Source: CAD feature listing. Evaluate the final solid. Frame: model axes, mm. A direction names the side the tool comes from. Coordinates: 2 decimals unless noted, no trailing zeros. Loops run counter-clockwise (first coordinate to the right, second up) from the corner with the lowest first, then second, coordinate; pieces in that order, holes last. Notation, with made-up numbers: (-32.75, -9) -> (-8.75, -9) arc R14 cw to (-8.75, 4) -> close; hole circle Ø9 at (24.5, -17). An arc over 180 degrees is marked (long way). Answer as CSV lines item,"result".
from build123d import *

# Parameters (mm, degrees)
SKETCH_2_W          = 210
SKETCH_2_H          = 100
EXTRUDE_1_DEPTH     = 130
SKETCH_3_W          = 200
SKETCH_3_H          = 90
CUT_EXTRUDE_1_DEPTH = 125
SKETCH_4_W          = 70
SKETCH_4_H          = 85
CUT_EXTRUDE_2_DEPTH = 125
CUT_EXTRUDE_4_DEPTH = 150
EXTRUDE_3_DEPTH     = 210
SKETCH_7_W          = 200
SKETCH_7_H          = 120
CUT_EXTRUDE_7_DEPTH = 35
EXTRUDE_6_DEPTH     = 4
EXTRUDE_7_DEPTH     = 4
SKETCH_13_W         = 192
SKETCH_13_H         = 52.689697424
CUT_EXTRUDE_9_DEPTH = 5


with BuildPart() as part:
    # 草图2 → 凸台-拉伸1 (new body)
    with BuildSketch(Plane.XY):
        Rectangle(SKETCH_2_W, SKETCH_2_H)
    extrude(amount=EXTRUDE_1_DEPTH)

    # 草图3 → 切除-拉伸1 (cut)
    with BuildSketch(Plane.XY):
        Rectangle(SKETCH_3_W, SKETCH_3_H)
    extrude(amount=CUT_EXTRUDE_1_DEPTH, mode=Mode.SUBTRACT)

    # 草图4 → 切除-拉伸2 (cut)
    with BuildSketch(Plane(origin=(0, 0, 0), x_dir=(1, 0, 0), z_dir=(0, 1, 0))):
        with Locations((0, -82.5)):
            Rectangle(SKETCH_4_W, SKETCH_4_H)
    extrude(amount=-CUT_EXTRUDE_2_DEPTH, mode=Mode.SUBTRACT)

    # 草图5 → 切除-拉伸4 (cut, symmetric)
    with BuildSketch(Plane(origin=(0, 0, 0), x_dir=(0, 0, -1), z_dir=(1, 0, 0))):
        with BuildLine():
            Line((0, 42), (0, -42))
            ThreePointArc((0, -42), (-61.900064838, 0), (0, 42))
        make_face()
    extrude(amount=CUT_EXTRUDE_4_DEPTH, both=True, mode=Mode.SUBTRACT)

    # 草图6 → 凸台-拉伸3 (add)
    with BuildSketch(Plane(origin=(105, 0, 0), x_dir=(0, 0, -1), z_dir=(1, 0, 0))):
        Polygon((-61.900064838, 50), (-61.900064838, 174.615745143), (-61.900064838, 180), (-21.900064838, 180), (-21.900064838, 50), align=None)
    extrude(amount=-EXTRUDE_3_DEPTH)

    # 草图7 → 切除-拉伸7 (cut)
    with BuildSketch(Plane.XY.offset(61.900064838)):
        with Locations((0, 115)):
            Rectangle(SKETCH_7_W, SKETCH_7_H)
    extrude(amount=-CUT_EXTRUDE_7_DEPTH, mode=Mode.SUBTRACT)

    # 草图11 → 凸台-拉伸6 (add)
    with BuildSketch(Plane(origin=(105, 0, 0), x_dir=(0, 0, -1), z_dir=(1, 0, 0))):
        Polygon((-130, 50), (-61.900064838, 180), (-61.900064838, 50), align=None)
    extrude(amount=-EXTRUDE_6_DEPTH)

    # 草图12 → 凸台-拉伸7 (add)
    with BuildSketch(Plane.ZY.offset(105)):
        Polygon((61.900064838, 180), (130, 50), (61.900064838, 50), align=None)
    extrude(amount=-EXTRUDE_7_DEPTH)

    # 草图13 → 切除-拉伸9 (cut)
    with BuildSketch(Plane(origin=(0, 50, 0), x_dir=(1, 0, 0), z_dir=(0, 1, 0))):
        with Locations((0, -98.24491355)):
            Rectangle(SKETCH_13_W, SKETCH_13_H)
    extrude(amount=-CUT_EXTRUDE_9_DEPTH, mode=Mode.SUBTRACT)


solid = part.part
(1) Cut plane B-B (x = -70). Return the cut outline in (y, z).
Computed values:
outline,"(-50, 0) -> (-45, 0) -> (-45, 12.47) arc R45.2 cw to (-45, 20.94) -> (-45, 125) -> (45, 125) -> (45, 124.59) -> (50, 124.59) -> (50, 130) -> (-50, 130) -> close; (45, 0) -> (50, 0) -> (50, 21.9) -> (180, 21.9) -> (180, 61.9) -> (175, 61.9) -> (175, 26.9) -> (55, 26.9) -> (55, 61.9) -> (50, 61.9) -> (50, 71.9) -> (45, 71.9) -> (45, 20.94) arc R45.2 cw to (45, 12.47) -> close"
(2) Access query for faces 4 (the flat face through (-8, 50, 71)), 5 (the flat face through (-1, 55, 45)), 6 (the flat face through (-100, -1, 84)), 7 (the flat face through (105, 67, 79)), 8 (the flat face through (-1, 50, 11)). Directions: +Z, -Z, +X, -X, +Y, -Y. A direction counts if a zero-diameter tool reaches every point of the face in a straight line with its end or side. Return the directions, or none.
Computed values:
face 4,"+Z, +Y"
face 5,"+Z"
face 6,"-Z"
face 7,"+Z, -Z, +X, +Y, -Y"
face 8,"-Z, +X, -X, +Y"
(3) Cut plane C-C (z = 111.5). Return the cut outline in (x, y).
Computed values:
outline,"(-105, -50) -> (-35, -50) -> (-35, -45) -> (-100, -45) -> (-100, 45) -> (-96, 45) -> (-96, 50) -> (-101, 50) -> (-101, 85.32) -> (-105, 85.32) -> close; (35, -50) -> (105, -50) -> (105, 85.32) -> (101, 85.32) -> (101, 50) -> (96, 50) -> (96, 45) -> (100, 45) -> (100, -45) -> (35, -45) -> close"
(4) Pin query (flat end, axial travel): pin 1 Ø1 at (x, y) = (-82.5, 74) entering from +Z; pin 2 Ø3 at (x, y) = (-19, -7) entering from -Z; pin 3 Ø1 at (x, z) = (2, 68) entering from -Y. Return the tip coordinate at first contact, or that it passes through.
Computed values:
pin 1,"z = 26.9"
pin 2,"z = 125"
pin 3,"y = 45"
(5) Material intervals for L1, parallel to Y at x = 43.5, z = 46; L2, parallel to X at y = 0, z = 98; L3, parallel to Z at x = -61, y = 49, sorted ascending. Write a range as [from, to].
Computed values:
L1,"[-50, -45], [45, 55], [175, 180]"
L2,"[-105, -100], [100, 105]"
L3,"[0, 71.9], [124.59, 130]"
(6) Cut plane A-A (x = 0.5). Return the cut outline in (y, z).
Computed values:
outline,"(-50, 0) -> (-45, 0) -> (-45, 12.47) arc R45.2 cw to (-45, 20.94) -> (-45, 40) -> (-50, 40) -> close; (-50, 125) -> (45, 125) -> (45, 124.59) -> (50, 124.59) -> (50, 130) -> (-50, 130) -> close; (45, 0) -> (50, 0) -> (50, 21.9) -> (180, 21.9) -> (180, 61.9) -> (175, 61.9) -> (175, 26.9) -> (55, 26.9) -> (55, 61.9) -> (50, 61.9) -> (50, 71.9) -> (45, 71.9) -> (45, 20.94) arc R45.2 cw to (45, 12.47) -> close"
(7) Cut plane D-D (y = 0). Return the cut outline in (x, z), then the cut area to 3 significant figures.
Computed values:
outline,"(-105, 61.9) -> (-100, 61.9) -> (-100, 125) -> (100, 125) -> (100, 61.9) -> (105, 61.9) -> (105, 130) -> (-105, 130) -> close"
area,"1,680 mm^2"
(8) Draft query along Y for faces 1 (the flat face through (-101, 87, 81)), 2 (the flat face through (-1, 45, 38)), 3 (the flat face through (103.028, 114.09, 96.427)). Return one class per face: released by +Y, released by -Y, zero draft, split by the parting line, or undercut.
Computed values:
face 1,"zero draft"
face 2,"undercut"
face 3,"released by +Y"
